Geometry check sheet. Reference: the model listing, model coordinates, mm. A direction names the side the tool comes from. Round coordinates to 2 decimals unless told otherwise and drop trailing zeros. Order: outer loops, then holes, each group sorted by start corner. A loop starts at its lowest first (then second) coordinate and runs counter-clockwise, first axis right, second up. Notation, with made-up numbers: (-22.5, 22.5) -> (22.5, 22.5) arc R25 ccw to (22.5, 46.5) -> close; hole circle Ø5 at (-13, -38.5). An arc over 180 degrees is marked (long way). Use a Markdown table: item, result. Add a question column.
Item 1: Material ranges on probe 1 along Y at (x, z) = (33, 0); probe 2 along X at (y, z) = (13.5, -8); probe 3 along Z at (x, y) = (-2, 4.75), recorded low to high. Write a range as [from, to].
Item 2: Sectioned sample at D-D, the plane y = -5. Record the cut outline in (x, z), and give its area (3 significant figures).
Item 3: Sectioned sample at B-B, the plane z = -11. Record the cut outline in (x, y).
Item 4: Sectioned sample at C-C, the plane x = 15.5. Record the cut outline in (y, z).
Item 5: Gauge pin test, flat ends, axial feed: pin 1 Ø1.5 at (x, z) = (27, -6.5) entering from +Y; pin 2 Ø10 at (y, z) = (3, 13) entering from -X; pin 3 Ø6 at (x, y) = (30.5, -2) entering from +Z. Record the tip position at first contact, or that the pin passes through.
Item 6: Sectioned sample at A-A, the plane y = 1.75. Record the cut outline in (x, z), and give its area (3 significant figures).
Item 7: Set-up check for faces 1 (the flat face through (10.47, 7.39, -6.03)), 2 (the flat face through (3.95, 7.39, 10.9)), 3 (the flat face through (-5.98, 7.39, 5.83)): record each of +Z, -Z, +X, -X, +Y, -Y from which the full face is reachable in a straight line by a thin tool's end or side.
Item 8: Mould release check, pull along X, two halves, no side actions. Record for faces 4 (the flat face through (-4.723, 7.388, -5.448)), 5 (the flat face through (13.81, 7.39, 0.75)), 6 (the flat face through (8.222, 7.388, -7.235)): pulls with the +X half, pulls with the -X half, needs draft (parallel to the pull), parting line crosses it, or undercut.
from build123d import *

# Parameters (mm, degrees)
F1_DEPTH = 8.89
F3_DEPTH = 23.876


with BuildPart() as f1:
    # F0 (on Front) → F1 (new body)
    with BuildSketch(Plane.XZ):
        with BuildLine():
            Line((8.2922062962, 18.3095482144), (5.8601442877, 19.2265168453))
            ThreePointArc((5.8601442877, 19.2265168453), (-20.0888672231, -0.6615548125), (7.1123886499, -18.7993129866))
            ThreePointArc((7.1123886499, -18.7993129866), (16.5371933279, -11.4245996827), (20.0997572392, 0))
            ThreePointArc((20.0997572392, 0), (16.8918852501, 10.8933215216), (8.2922062962, 18.3095482144))
        make_face()
        with BuildLine():
            ThreePointArc((20.0997572392, 0), (16.5371933279, -11.4245996827), (7.1123886499, -18.7993129866))
            Line((7.1123886499, -18.7993129866), (41.7047212119, -5.7119138))
            ThreePointArc((41.7047212119, -5.7119138), (33.4467243991, 0), (41.7047212119, 5.7119138))
            Line((41.7047212119, 5.7119138), (8.2922062962, 18.3095482144))
            ThreePointArc((8.2922062962, 18.3095482144), (16.8918852501, 10.8933215216), (20.0997572392, 0))
        make_face()
        with BuildLine():
            ThreePointArc((41.7047212119, 5.7119138), (33.4467243991, 0), (41.7047212119, -5.7119138))
            Line((41.7047212119, -5.7119138), (41.7047212119, 5.7119138))
        make_face()
        with BuildLine():
            Line((41.7047212119, 5.7119138), (41.7047212119, -5.7119138))
            ThreePointArc((41.7047212119, -5.7119138), (44.5716087418, -3.4725723137), (45.6555533566, 0))
            ThreePointArc((45.6555533566, 0), (44.5716087418, 3.4725723137), (41.7047212119, 5.7119138))
        make_face()
    extrude(amount=F1_DEPTH)

    # F2 (on face) → F3 (join)
    with BuildSketch(Plane.XZ.offset(8.89)):
        Polygon((5.8601442877, 14.4999762997), (1.981993678, 7.1901451267), (7.8095722297, 5.8180000225), align=None)
        Polygon((7.8095722297, 5.8180000225), (1.981993678, 7.1901451267), (-1.1140019774, 1.3545786852), (5.1359782959, -4.3957886373), (9.519282463, -1.7963689762), align=None)
        Polygon((1.981993678, 7.1901451267), (-10.7028093189, 10.1768728346), (-1.1140019774, 1.3545786852), align=None)
        Polygon((5.1359782959, -4.3957886373), (-1.1140019774, 1.3545786852), (-8.434349671, -12.4433655292), align=None)
        Polygon((9.519282463, -1.7963689762), (5.1359782959, -4.3957886373), (11.3962469622, -10.1556219161), align=None)
        Polygon((18.2240977883, 3.365825396), (7.8095722297, 5.8180000225), (9.519282463, -1.7963689762), align=None)
    extrude(amount=-F3_DEPTH)


solid = f1.part
Found:
| question | item | result |
|---|---|---|
| 1 | probe 1 | y = [-8.89, 0] |
| 1 | probe 2 | x = [-6.08, -0.94], [9.05, 10.91] |
| 1 | probe 3 | z = [-8.63, -0.32], [2.17, 8.13] |
| 2 | outline | (5.86, 19.23) arc R20.1 ccw (long way) to (7.11, -18.8) -> (41.7, -5.71) arc R6.1 ccw to (41.7, 5.71) -> close |
| 2 | area | 1,790 mm2 |
| 3 | outline | (-16.82, -8.89) -> (27.73, -8.89) -> (27.73, 0) -> (-6, 0) -> (-6, 14.99) -> (-7.67, 14.99) -> (-7.67, 0) -> (-16.82, 0) -> close |
| 4 | outline | (-8.89, -15.63) -> (0, -15.63) -> (0, 1.75) -> (14.99, 1.75) -> (14.99, 4.01) -> (0, 4.01) -> (0, 15.59) -> (-8.89, 15.59) -> close |
| 5 | pin 1 | stops at y = 0 |
| 5 | pin 2 | stops at x = -17.97 |
| 5 | pin 3 | stops at z = 11.07 |
| 6 | outline | (-10.7, 10.18) -> (-1.11, 1.35) -> (-8.43, -12.44) -> (5.14, -4.4) -> (11.4, -10.16) -> (9.52, -1.8) -> (18.22, 3.37) -> (7.81, 5.82) -> (5.86, 14.5) -> (1.98, 7.19) -> close |
| 6 | area | 266 mm2 |
| 7 | face 1 | +X, +Y |
| 7 | face 2 | +Z, +Y |
| 7 | face 3 | -X, +Y |
| 8 | face 4 | pulls with the -X half |
| 8 | face 5 | pulls with the +X half |
| 8 | face 6 | undercut |
